Source: CAD feature listing. Evaluate the final solid. Frame: model axes, mm. A direction names the side the tool comes from. Round coordinates to 2 decimals unless told otherwise and drop trailing zeros. Write each loop counter-clockwise with the first axis right and the second up, starting at its lowest first coordinate (ties: lowest second). Pieces come first, ordered by that corner, then holes. Notation, with made-up numbers: (55, 15.25) -> (68, 15.25) arc R6 cw to (68, 24.25) -> close; hole circle Ø4 at (26, 62). An arc over 180 degrees is marked (long way). Put each result on its own line as item: value.
Autodesk Fusion 360 part; units mm, degrees
sketch "Sketch1" plane through (0, 0, 0) normal (0, 0, 1) x (1, 0, 0)
  line L0 (9.5, 29) -> (9.5, 22) construction
  line L1 (9.5, 0) -> (9.5, -3) construction
  line L2 (9.5, -3) -> (13.5, -3)
  line L3 (9.5, -3) -> (5.5, -3)
  line L4 (4.5, -2) -> (4.5, 0)
  line L5 (14.5, -2) -> (14.5, 0)
  line L6 (15, 0) -> (14.5, 0)
  line L7 (4.5, 0) -> (4, 0)
  line L8 (13.3, 22.5) -> (13.3, 27)
  line L9 (5.7, 22.5) -> (5.7, 27)
  line L10 (11.3, 29) -> (7.7, 29)
  line L11 (19, 4) -> (19, 18)
  line L12 (0, 4) -> (0, 18)
  arc A0 (0, 4) -> (4, 0) centre (4, 4) ccw
  arc A1 (15, 0) -> (19, 4) centre (15, 4) ccw
  arc A2 (19, 18) -> (15, 22) centre (15, 18) ccw
  arc A3 (4, 22) -> (0, 18) centre (4, 18) ccw
  line L13 (15, 22) -> (13.8, 22)
  arc A4 (13.3, 22.5) -> (13.8, 22) centre (13.8, 22.5) ccw
  line L14 (4, 22) -> (5.2, 22)
  arc A5 (5.2, 22) -> (5.7, 22.5) centre (5.2, 22.5) ccw
  arc A6 (13.3, 27) -> (11.3, 29) centre (11.3, 27) ccw
  arc A7 (7.7, 29) -> (5.7, 27) centre (7.7, 27) ccw
  arc A8 (13.5, -3) -> (14.5, -2) centre (13.5, -2) ccw
  arc A9 (4.5, -2) -> (5.5, -3) centre (5.5, -2) ccw
  point P0 (19, 0)
  point P1 (13.3, 22)
  dimension "d1" = 19
  dimension "d6" = 3.8
  dimension "d8" = 4
  dimension "d9" = 4
  dimension "d10" = 4
  dimension "d11" = 4
  dimension "d12" = 0.5
  dimension "d13" = 0.5
  dimension "d14" = 2
  dimension "d15" = 2
  dimension "d16" = 1
  dimension "d17" = 1
extrude "Extrude1" add sketch "Sketch1" along normal blind 2
sketch "Sketch2" plane through (13.3, 0, 0) normal (1, 0, 0) x (0, 1, 0)
  line L0 (22.5, 0) -> (27, 0)
  line L1 (27, 0) -> (27, 2)
  line L2 (27, 2) -> (22.5, 2)
  line L3 (22.5, 2) -> (22.5, 0)
  line L4 (27, 1) -> (22.5, 1) construction
  circle A0 centre (26.2099, 1) radius 0.65
  dimension "d20" = 1.3
extrude "Extrude2" cut sketch "Sketch2" against normal blind 20 contours A0
Q1. Reachability of faces 1 (the flat face through (13.3, 25, 1)), 2 (the flat face through (19, 11, 1)), 3 (the flat face through (10, 29, 1)), 4 (the flat face through (4.5, -1, 1)), 5 (the flat face through (5, 22, 1)) from +Z, -Z, +X, -X, +Y, -Y: full face, straight path, thin tool, end or side. Return the list, or none.
Ans:
face 1: +Z, -Z, +X, +Y
face 2: +Z, -Z, +X, +Y, -Y
face 3: +Z, -Z, +X, -X, +Y
face 4: +Z, -Z, -X, -Y
face 5: +Z, -Z, -X, +Y
Q2. Pin query (flat end, axial travel): pin 1 (0.6 mm diameter, centred on y = -1.5, z = 1, fed in from -X); pin 2 (0.6 mm diameter, centred on y = 24, z = 1, fed in from +X); pin 3 (1 mm diameter, centred on x = 14.5, z = 1, fed in from +Y). Return the tip coordinate at first contact, or that it passes through.
Ans:
pin 1: stops at x = 4.5
pin 2: stops at x = 13.3
pin 3: stops at y = 22
Q3. Cut plane A-A on z = 1. Output: boundary loops of the cut face in (x, y).
Ans:
outline: (0, 4) arc R4 ccw to (4, 0) -> (4.5, 0) -> (4.5, -2) arc R1 ccw to (5.5, -3) -> (13.5, -3) arc R1 ccw to (14.5, -2) -> (14.5, 0) -> (15, 0) arc R4 ccw to (19, 4) -> (19, 18) arc R4 ccw to (15, 22) -> (13.8, 22) arc R0.5 cw to (13.3, 22.5) -> (13.3, 25.56) -> (5.7, 25.56) -> (5.7, 22.5) arc R0.5 cw to (5.2, 22) -> (4, 22) arc R4 ccw to (0, 18) -> close; (5.7, 26.86) -> (13.3, 26.86) -> (13.3, 27) arc R2 ccw to (11.3, 29) -> (7.7, 29) arc R2 ccw to (5.7, 27) -> close
Q4. Material intervals for line 1 (Y direction, x = 15, z = 0.3); line 2 (X direction, y = 23, z = 0.2); line 3 (Y direction, x = 14.25, z = 1.6), sorted ascending. Write a range as [from, to].
Ans:
line 1: y = [0, 22]
line 2: x = [5.7, 13.3]
line 3: y = [-2.66, 22]
Q5. Draft query along Z for faces 6 (the cylindrical face through (1.141, 20.797, 0.986)), 7 (the flat face through (9, 13, 0)), 8 (the cylindrical face through (9.55, 25.56, 1.03)). Return one class per face: +Z half, -Z half, draft (parallel to the pull), parting line (faces both ways), or undercut.
Ans:
face 6: draft
face 7: -Z half
face 8: undercut
Q6. Cut plane B-B on y = 20. Output: boundary loops of the cut face in (x, z), and give its area (3 significant figures).
Ans:
outline: (0.54, 0) -> (18.46, 0) -> (18.46, 2) -> (0.54, 2) -> close
area: 35.9 mm^2
